```python
from build123d import *

# Parameters (mm, degrees)
SKETCH1_W           = 70
SKETCH1_H           = 70
BOSS_EXTRUDE1_DEPTH = 120
SKETCH2_R           = 25
BOSS_EXTRUDE2_DEPTH = 40
SKETCH3_R           = 30
BOSS_EXTRUDE3_DEPTH = 10
SKETCH4_R           = 25
BOSS_EXTRUDE4_DEPTH = 70
SKETCH5_R           = 25
BOSS_EXTRUDE5_DEPTH = 20
BOSS_EXTRUDE6_DEPTH = 35
CUT_EXTRUDE1_DEPTH  = 25
SKETCH9_R           = 20
BOSS_EXTRUDE7_DEPTH = 50


with BuildPart() as part:
    # Sketch1 → Boss-Extrude1 (new body)
    with BuildSketch(Plane(origin=(0, 0, 0), x_dir=(1, 0, 0), z_dir=(0, 1, 0))):
        Rectangle(SKETCH1_W, SKETCH1_H)
    extrude(amount=BOSS_EXTRUDE1_DEPTH)

    # Sketch2 → Boss-Extrude2 (add)
    with BuildSketch(Plane.XZ):
        with Locations(Location((0, 0, 0), (0, 0, 270))):
            Circle(SKETCH2_R)
    extrude(amount=BOSS_EXTRUDE2_DEPTH)

    # Sketch3 → Boss-Extrude3 (add)
    with BuildSketch(Plane.XZ.offset(40)):
        with Locations(Location((0, 0, 0), (0, 0, 270))):
            Circle(SKETCH3_R)
    extrude(amount=BOSS_EXTRUDE3_DEPTH)

    # Sketch4 → Boss-Extrude4 (add)
    with BuildSketch(Plane.XY.offset(35)):
        with BuildLine():
            Line((65, 114.048192782), (35, 120))
            Line((35, 120), (35, 35.50717312))
            ThreePointArc((35, 35.50717312), (107.037756153, 52.991198743), (65, 114.048192782))
        make_face()
        with Locations((65, 69.048192782)):
            Circle(SKETCH4_R, mode=Mode.SUBTRACT)
    extrude(amount=-BOSS_EXTRUDE4_DEPTH)

    # Sketch5 → Boss-Extrude5 (add)
    with BuildSketch(Plane.XZ.offset(50)):
        with Locations(Location((0, 0, 0), (0, 0, 270))):
            Circle(SKETCH5_R)
    extrude(amount=BOSS_EXTRUDE5_DEPTH)

    # Sketch6 → Boss-Extrude6 (add, symmetric)
    with BuildSketch(Plane(origin=(0, 0, 0), x_dir=(0, 0, -1), z_dir=(1, 0, 0))):
        with BuildLine():
            ThreePointArc((-35, -190), (0, -225), (35, -190))
            Line((35, -190), (35, -155))
            Line((35, -155), (35, -70))
            Line((35, -70), (-35, -70))
            Line((-35, -70), (-35, -155))
            Line((-35, -155), (-35, -190))
        make_face()
    extrude(amount=BOSS_EXTRUDE6_DEPTH, both=True)

    # Sketch8 → Cut-Extrude1 (cut, symmetric)
    with BuildSketch(Plane(origin=(0, 0, 0), x_dir=(0, 0, -1), z_dir=(1, 0, 0))):
        with BuildLine():
            Line((-35, -130), (-35, -190))
            ThreePointArc((-35, -190), (0, -225), (35, -190))
            Line((35, -190), (35, -130))
            Line((35, -130), (-35, -130))
        make_face()
    extrude(amount=CUT_EXTRUDE1_DEPTH, both=True, mode=Mode.SUBTRACT)

    # Sketch9 → Boss-Extrude7 (add)
    with BuildSketch(Plane(origin=(-25, 0, 0), x_dir=(0, 0, -1), z_dir=(1, 0, 0))):
        with Locations((0, -190)):
            Circle(SKETCH9_R)
    extrude(amount=BOSS_EXTRUDE7_DEPTH)


solid = part.part
```
Work out the finished part from the listing and answer in its coordinate system (mm). A direction names the side the tool comes from. Coordinates: 2 decimals unless noted, no trailing zeros. Write each loop counter-clockwise with the first axis right and the second up, starting at its lowest first coordinate (ties: lowest second). Pieces come first, ordered by that corner, then holes.
Q1. A cutting plane is placed at A-A, the plane x = 0. Give the vertices of the cut face in (y, z).
Q2. A cutting plane is placed at B-B, the plane z = 16.5. State how many separate pieces and enclosed holes the cut face has, then the cut area to 3 significant figures.
Q3. Find the intervals of material crossed by line 1 (Y direction, x = 65, z = -8); line 2 (X direction, y = -203.5, z = 30.5); line 3 (Y direction, x = 5.5, z = 1), in increasing order.
Q4. Each of these flat-tipped pins is pushed along its axis until it touches: pin 1 Ø15 at (x, z) = (-7.5, -7) entering from -Y; pin 2 Ø3 at (y, z) = (52, 18) entering from +X; pin 3 Ø2 at (x, y) = (-17.5, -17.5) entering from +Z. Where does it stop, or does it pass through?
Q5. Which of the six approach directions +Z, -Z, +X, -X, +Y, -Y give full straight-line access (tool end or side, diameter ignored) to faces 4 (the face through (35, -146, 0)), 5 (the face through (0, -130, 0)), 6 (the face through (35, 18, 0)), 7 (the face through (-25, -166, 0))?
Q6. Determine the mould class of faces 1 (the face through (0, -116, 35)), 2 (the face through (24, -70, -8)), 3 (the face through (-29.93, -224.99, 0.77)) for opening direction Y: released by +Y, released by -Y, zero draft, split by the parting line, or undercut.
Q7. A cutting plane is placed at D-D, the plane y = -96. Give the vertices of the cut face in (x, z).
Q8. A cutting plane is placed at C-C, the plane x = 15. Give the vertices of the cut face in (y, z), then the cut area to 3 significant figures.
Findings below:
1. outline: circle Ø40 at (-190, 0); (-130, -35) - (-70, -35) - (-70, -25) - (-50, -25) - (-50, -30) - (-40, -30) - (-40, -25) - (0, -25) - (0, -35) - (120, -35) - (120, 35) - (0, 35) - (0, 25) - (-40, 25) - (-40, 30) - (-50, 30) - (-50, 25) - (-70, 25) - (-70, 35) - (-130, 35) - close
2. separate pieces: 1
2. enclosed holes: 2
2. area: 22,200 mm2
3. line 1: y = 24.05 to 44.05, 94.05 to 114.05
3. line 2: x = -35 to -25, 25 to 35
3. line 3: y = -209.97 to -170.03, -130 to 120
4. pin 1: stops at y = -210
4. pin 2: stops at x = 107.23
4. pin 3: stops at z = 18.78
5. face 4: +Z, -Z, +X, -Y
5. face 5: +Z, -Z
5. face 6: +Z, -Z, -Y
5. face 7: none
6. face 1: zero draft
6. face 2: undercut
6. face 3: released by -Y
7. outline: (-35, -35) - (35, -35) - (35, 35) - (-35, 35) - close
8. outline: circle Ø40 at (-190, 0); (-130, -35) - (-70, -35) - (-70, -20) - (-50, -20) - (-50, -25.98) - (-40, -25.98) - (-40, -20) - (0, -20) - (0, -35) - (120, -35) - (120, 35) - (0, 35) - (0, 20) - (-40, 20) - (-40, 25.98) - (-50, 25.98) - (-50, 20) - (-70, 20) - (-70, 35) - (-130, 35) - close
8. area: 16,800 mm2
